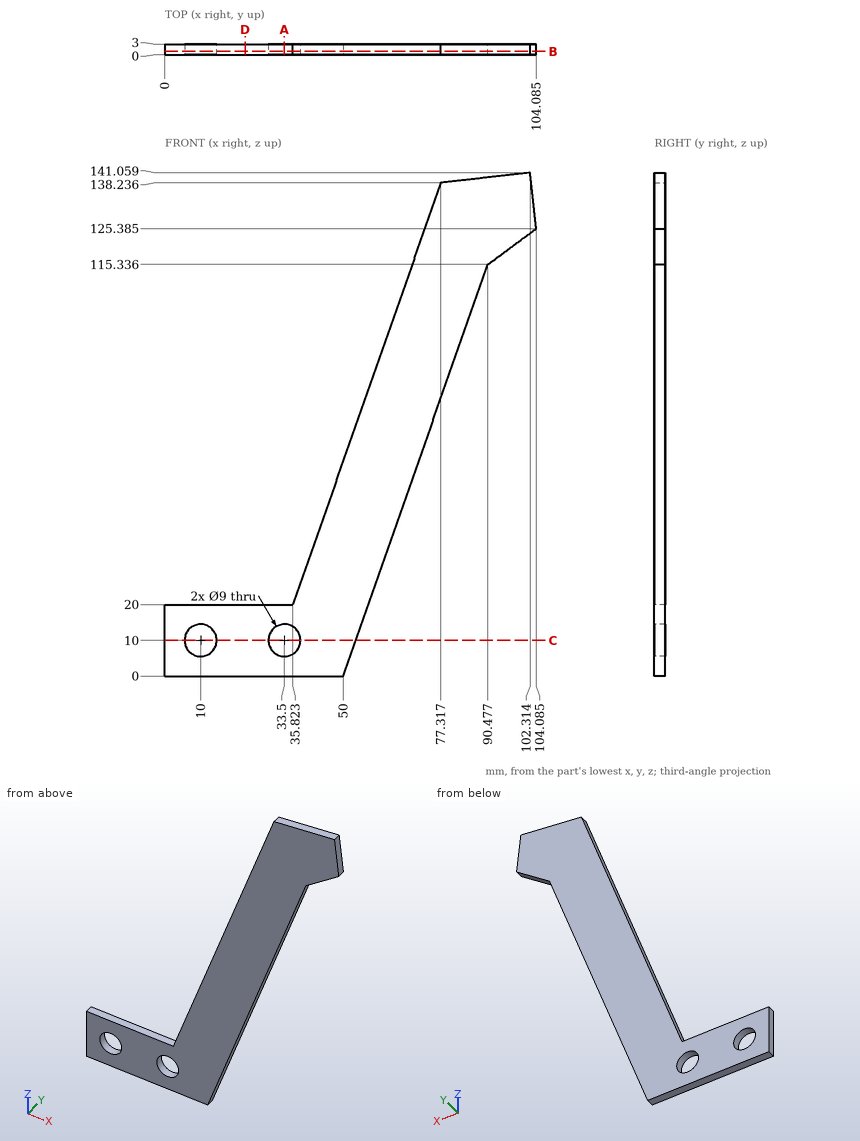
Could you check a few things on this drawing? It's one solid part, dimensions in mm from its lowest x, y, z. Give positions to 0.01 mm unless a question says otherwise; leave off trailing zeros. Order: outer loops, then holes, each group sorted by start corner. A loop starts at its lowest first (then second) coordinate and runs counter-clockwise, first axis right, second up. Notation, with made-up numbers: M 22,54.25 L 62,54.25 A18 cw 62,71.25 Z; hole C -5.75,50.5 d9. An arc over 180 degrees is marked long. Use one line per item in the form item = value. Start each with the question number.
Item 1: If I drill on line 1 along Z through (x, y) = (10, 2.3); line 2 along Z through (x, y) = (17, 1.9); line 3 along X through (y, z) = (2.95, 14) (1 decimal), over which ranges is the centre line in solid material (lowest first)?
Item 2: If we section it at C-C (z = 10): Write out the boundary of the cut face in (x, y).
Item 3: If we section it at A-A (x = 33.5): Write out the boundary of the cut face in (y, z).
Item 4: If we section it at D-D (x = 22.5): Write out the boundary of the cut face in (y, z), then the cut area to 3 significant figures.
Item 5: If we section it at B-B (y = 0.95): Write out the boundary of the cut face in (x, z) (1 decimal).
Item 6: Will these pins go through, and if not, where does the flat tip stop? pin 1 Ø11.5 at (x, z) = (33.5, 10) entering from -Y; pin 2 Ø1.5 at (x, y) = (10.5, 1.5) entering from +Z.
Outcome:
q1.line_1 = 0 to 5.5, 14.5 to 20
q1.line_2 = 0 to 20
q1.line_3 = 0 to 7.9, 12.1 to 31.4, 35.6 to 54.9
q2.outline = M 0,0 L 5.5,0 L 5.5,3 L 0,3 Z; M 14.5,0 L 29,0 L 29,3 L 14.5,3 Z; M 38,0 L 53.51,0 L 53.51,3 L 38,3 Z
q3.outline = M 0,0 L 3,0 L 3,5.5 L 0,5.5 Z; M 0,14.5 L 3,14.5 L 3,20 L 0,20 Z
q4.outline = M 0,0 L 3,0 L 3,20 L 0,20 Z
q4.area = 60.0 mm2
q5.outline = M 0,0 L 50,0 L 90.5,115.3 L 104.1,125.4 L 102.3,141.1 L 77.3,138.2 L 35.8,20 L 0,20 Z; hole C 10,10 d9; hole C 33.5,10 d9
q6.pin_1 = 0
q6.pin_2 = 20
